Can you work these out from the model? Positions are in its coordinate system, mm. A direction names the side the tool comes from. Give positions to 0.01 mm unless a question says otherwise; leave off trailing zeros. Order: outer loops, then holes, each group sorted by start corner. A loop starts at its lowest first (then second) coordinate and runs counter-clockwise, first axis right, second up. Notation, with made-up numbers: (67.25, 47) - (121.25, 47) arc R36 ccw to (121.25, 83) - close; hole circle Ø8 at (28, 52.5). An arc over 180 degrees is marked (long way). Answer as CSV lines item,"result".
```python
from build123d import *

# Parameters (mm, degrees)
F0_W     = 95.1874652
F0_H     = 21.3499954
F0_R     = 6.7062477
F1_DEPTH = 1.5875
F2_R     = 10.6749977
F4_DEPTH = 12
F5_R     = 2.2479
F5_R_2   = 3.175
F6_DEPTH = 13.5875
F7_R     = 3.96875
F8_DEPTH = 7.2375014


with BuildPart() as f1:
    # F0 (on Top) → F1 (new body)
    with BuildSketch(Plane.XY):
        with Locations((47.5937326, -10.6749977)):
            Rectangle(F0_W, F0_H)
        with Locations((10.6749977, -10.6749977)):
            Circle(F0_R, mode=Mode.SUBTRACT)
        with Locations((84.5124675, -10.6749977)):
            Circle(F0_R, mode=Mode.SUBTRACT)
    extrude(amount=F1_DEPTH)

    # F2
    f2_edges = [f1.edges().sort_by_distance(p)[0] for p in [
        (0, 0, 0.79375),
        (95.187465, 0, 0.79375),
    ]]
    fillet(f2_edges, radius=F2_R)

    # F3 (on face) → F4 (join)
    with BuildSketch(Plane.XY.offset(1.5875)):
        with BuildLine():
            Line((4.5476495872, -14.9999954), (0, -14.9999954))
            Line((0, -14.9999954), (0, -21.3499954))
            Line((0, -21.3499954), (95.1874652, -21.3499954))
            Line((95.1874652, -21.3499954), (95.1874652, -14.9999954))
            Line((95.1874652, -14.9999954), (90.6398156128, -14.9999954))
            ThreePointArc((90.6398156128, -14.9999954), (84.5124675, -18.1749977), (78.3851193872, -14.9999954))
            Line((78.3851193872, -14.9999954), (16.8023458128, -14.9999954))
            ThreePointArc((16.8023458128, -14.9999954), (10.6749977, -18.1749977), (4.5476495872, -14.9999954))
        make_face()
        with BuildLine():
            Line((0, -10.6749977), (0, -14.9999954))
            Line((0, -14.9999954), (4.5476495872, -14.9999954))
            ThreePointArc((4.5476495872, -14.9999954), (8.4061996532, -3.5263925617), (18.1749977, -10.6749977))
            ThreePointArc((18.1749977, -10.6749977), (17.8236028383, -12.9437957468), (16.8023458128, -14.9999954))
            Line((16.8023458128, -14.9999954), (78.3851193872, -14.9999954))
            ThreePointArc((78.3851193872, -14.9999954), (82.2436694532, -3.5263925617), (92.0124675, -10.6749977))
            ThreePointArc((92.0124675, -10.6749977), (91.6610726383, -12.9437957468), (90.6398156128, -14.9999954))
            Line((90.6398156128, -14.9999954), (95.1874652, -14.9999954))
            Line((95.1874652, -14.9999954), (95.1874652, -10.6749977))
            ThreePointArc((95.1874652, -10.6749977), (92.0608307628, -3.1266344372), (84.5124675, 0))
            Line((84.5124675, 0), (10.6749977, 0))
            ThreePointArc((10.6749977, 0), (3.1266344372, -3.1266344372), (0, -10.6749977))
        make_face()
    extrude(amount=F4_DEPTH)

    # F5 (on face) → F6 (cut, through all)
    with BuildSketch(Plane.XY.offset(13.5875)):
        with Locations((51.0505421177, -10.6749977)):
            Circle(F5_R)
        with Locations((63.0499501, -7.6956285)):
            Circle(F5_R_2)
        with Locations((25.3187477, -10.6749977)):
            Circle(F5_R)
    extrude(amount=-F6_DEPTH, mode=Mode.SUBTRACT)

    # F7 (on face) → F8 (cut)
    with BuildSketch(Plane(origin=(0, 0, 0), x_dir=(1, 0, 0), z_dir=(0, 0, -1))):
        with Locations((51.0505421177, 10.6749977)):
            Circle(F7_R)
        with Locations((25.3187477, 10.6749977)):
            Circle(F7_R)
    extrude(amount=-F8_DEPTH, mode=Mode.SUBTRACT)


solid = f1.part
```
1) Which directions (+Z, -Z, +X, -X, +Y, -Y) give clear straight access to the entire face, cutting with the end or side of a thin tool? Please do faces 4 (the flat face through (53, -9, 7.238)), 5 (the cylindrical face through (16.87, -13.24, 0.78)), 6 (the flat face through (79, -15, 1.588)).
Answer block:
face 4,"-Z"
face 5,"+Z, -Z"
face 6,"+Z"
2) I'm going to push flat-ended pins straight in: P1, Ø4, axis at y = -8.5, z = 8.5, coming from the +X side; P2, Ø5, axis at y = -3, z = 3, coming from the +X side; P3, Ø1, axis at y = -8.5, z = 5, coming from the +X side. Where does each tip first touch, or does it pass through?
Answer block:
P1,"x = 95.19"
P2,"x = 93.85"
P3,"x = 95.06"
3) I want a section at D-D on y = -1.75. Write out the boundary of the cut face in (x, z).
Answer block:
outline,"(4.82, 0) - (90.37, 0) - (90.37, 13.59) - (4.82, 13.59) - close"
4) I need wall thicknesses on line 1 along X through (y, z) = (-11, 5); line 2 along Y through (x, z) = (63, 11); line 3 along Y through (x, z) = (51, 1.25). Which ranges of each line are inside material? Lowest first, please. Write a range as [from, to].
Answer block:
line 1,"[0, 3.18], [18.17, 21.36], [29.27, 47.1], [55.01, 77.02], [92.01, 95.19]"
line 2,"[-21.35, -10.87], [-4.52, 0]"
line 3,"[-21.35, -14.64], [-6.71, 0]"
5) If we mould it in two halves opening along Y, with no side actions, what happens to faces 1 (the flat face through (95.187, -16, 7)), 2 (the cylindrical face through (27.463, -10, 10.457)), 3 (the flat face through (47, -21.35, 7))? For each: +Y half, -Y half, draft (parallel to the pull), parting line (faces both ways), or undercut.
Answer block:
face 1,"draft"
face 2,"undercut"
face 3,"-Y half"
6) I want a section at A-A on y = -16.25. Write out the boundary of the cut face in (x, z), plus the area to 3 significant figures.
Answer block:
outline,"(0, 0) - (6.95, 0) - (6.95, 1.59) - (5.66, 1.59) - (5.66, 13.59) - (0, 13.59) - close; (14.4, 0) - (80.79, 0) - (80.79, 1.59) - (79.5, 1.59) - (79.5, 13.59) - (15.69, 13.59) - (15.69, 1.59) - (14.4, 1.59) - close; (88.24, 0) - (95.19, 0) - (95.19, 13.59) - (89.53, 13.59) - (89.53, 1.59) - (88.24, 1.59) - close"
area,"1,030 mm2"
7) I want a section at B-B on x = 80. Write out the boundary of the cut face in (y, z).
Answer block:
outline,"(-21.35, 0) - (-15.64, 0) - (-15.64, 1.59) - (-16.67, 1.59) - (-16.67, 13.59) - (-21.35, 13.59) - close; (-5.71, 0) - (0, 0) - (0, 13.59) - (-4.68, 13.59) - (-4.68, 1.59) - (-5.71, 1.59) - close"
8) I want a section at C-C on z = 11. Write out the boundary of the cut face in (x, y) (3 decimals).
Answer block:
outline,"(0, -21.35) - (95.187, -21.35) - (95.187, -10.675) arc R10.675 ccw to (84.512, 0) - (10.675, 0) arc R10.675 ccw to (0, -10.675) - close; hole circle Ø15 at (10.675, -10.675); hole circle Ø4.496 at (25.319, -10.675); hole circle Ø4.496 at (51.051, -10.675); hole circle Ø6.35 at (63.05, -7.696); hole circle Ø15 at (84.512, -10.675)"
